Source: three-view drawing plus pictorial views. Frame: mm from the lowest corner of the part. Coordinates: 2 decimals unless noted, no trailing zeros. Write each loop counter-clockwise with the first axis right and the second up, starting at its lowest first coordinate (ties: lowest second). Pieces come first, ordered by that corner, then holes. Notation, with made-up numbers: M -35.5,46 L 9.5,46 A21 ccw 9.5,53 Z; hole C 61,44.25 d1. An arc over 180 degrees is marked long. Use CSV: the item, a comma, the result in double quotes.
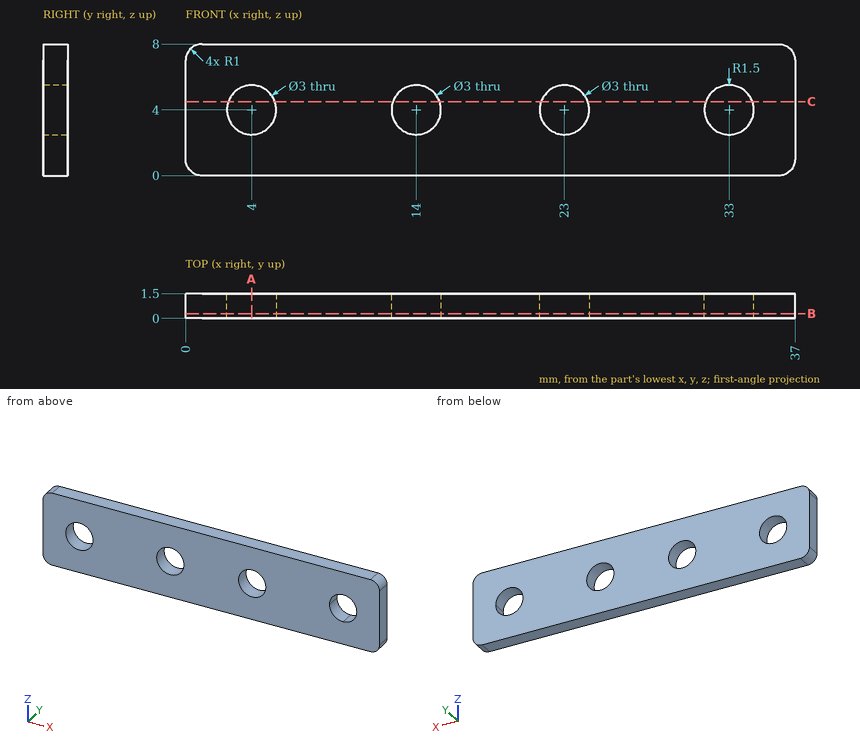
1. Material intervals for line 1 (X direction, y = 1.05, z = 4); line 2 (Z direction, x = 4, y = 0.4); line 3 (X direction, y = 0.75, z = 4.75), sorted ascending. Write a range as [from, to].
Resolved:
line 1,"x = [0, 2.5], [5.5, 12.5], [15.5, 21.5], [24.5, 31.5], [34.5, 37]"
line 2,"z = [0, 2.5], [5.5, 8]"
line 3,"x = [0, 2.7], [5.3, 12.7], [15.3, 21.7], [24.3, 31.7], [34.3, 37]"
2. Section B-B (y = 0.3). Return loops of the section in (x, z), then the cut area to 3 significant figures.
Resolved:
outline,"M 0,1 A1 ccw 1,0 L 36,0 A1 ccw 37,1 L 37,7 A1 ccw 36,8 L 1,8 A1 ccw 0,7 Z; hole C 4,4 d3; hole C 14,4 d3; hole C 23,4 d3; hole C 33,4 d3"
area,"267 mm^2"
3. Section C-C (z = 4.5). Return loops of the section in (x, y).
Resolved:
outline,"M 0,0 L 2.59,0 L 2.59,1.5 L 0,1.5 Z; M 5.41,0 L 12.59,0 L 12.59,1.5 L 5.41,1.5 Z; M 15.41,0 L 21.59,0 L 21.59,1.5 L 15.41,1.5 Z; M 24.41,0 L 31.59,0 L 31.59,1.5 L 24.41,1.5 Z; M 34.41,0 L 37,0 L 37,1.5 L 34.41,1.5 Z"
4. Section A-A (x = 4). Return loops of the section in (y, z).
Resolved:
outline,"M 0,0 L 1.5,0 L 1.5,2.5 L 0,2.5 Z; M 0,5.5 L 1.5,5.5 L 1.5,8 L 0,8 Z"
5. Contact query for a flat-ended pin moving along its axis: pin 1 Ø1.8 at (x, z) = (14, 4) entering from -Y. Output: stop coordinate, or through.
Resolved:
pin 1,"passes through"
